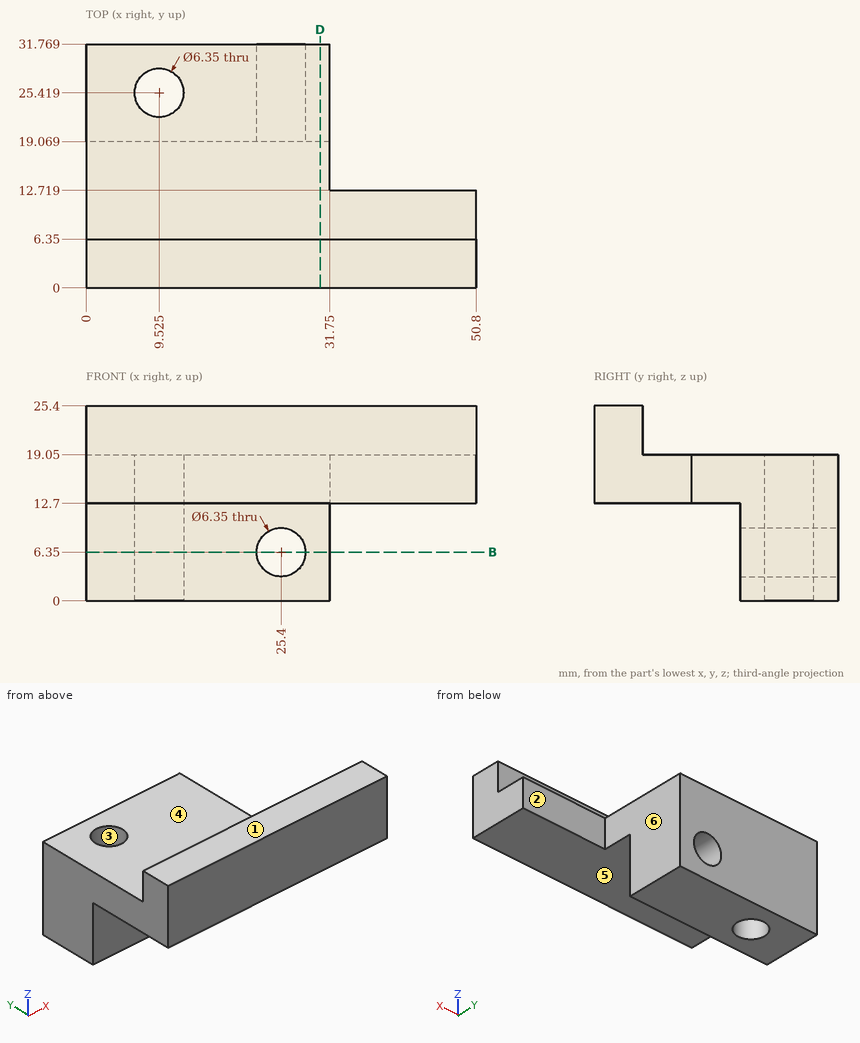
Check sheet for the drawn part. Datum: minimum x, y, z corner. Units: mm. A direction names the side the tool comes from. Give positions to 0.01 mm unless a question says otherwise; leave off trailing zeros. Loops run counter-clockwise (first coordinate to the right, second up) from the corner with the lowest first, then second, coordinate; pieces in that order, holes last. Notation, with made-up numbers: (30, -38) - (58, -38) arc R35 ccw to (58, -6) - close; hole circle Ø4 at (-36.5, 32.25). An arc over 180 degrees is marked (long way). Write each question's results on one line, items separated by ' | '.
1) Depth check by flat-ended pin: P1, Ø3, axis at x = 10.5, y = 25.5, coming from the +Z side; P2, Ø4, axis at x = 13.5, z = 2.5, coming from the -Y side; P3, Ø15.5, axis at x = 19.5, y = 8, coming from the -Z side; P4, Ø7, axis at x = 30, z = 23, coming from the +Y side. Enter the tip coordinate at first touch or a pass-through.
Solution:
P1: through | P2: y = 19.07 | P3: z = 12.7 | P4: y = 6.35
2) Sectioned sample at B-B on z = 6.35. Count the separate pieces of the cut face and the enclosed holes in it, plus the area to 3 significant figures.
Solution:
separate pieces: 2 | enclosed holes: 1 | area: 291 mm2
3) Tool access check on the marked faces 4, 5 and 6. Record the directions out of +Z, -Z, +X, -X, +Y, -Y that give a thin tool (end or side, any length) a straight path to the whole face; none if there is none.
Solution:
face 4: +Z, +X, -X, +Y | face 5: -Z, +X, -X, -Y | face 6: +Z, -Z, +X, +Y
4) Material ranges on L1, parallel to Z at x = 30.5, y = 19; L2, parallel to Y at x = 31, z = 19.5; L3, parallel to X at y = 22, z = 5.75, recorded low to high. Write a range as from..to.
Solution:
L1: 12.7..19.05 | L2: 0..6.35 | L3: 0..22.28, 28.52..31.75
5) Mould release check, pull along Y, two halves, no side actions. Record for the marked faces 1, 2 and 3: pulls with the +Y half, pulls with the -Y half, needs draft (parallel to the pull), parting line crosses it, or undercut.
Solution:
face 1: needs draft | face 2: pulls with the +Y half | face 3: undercut
6) Sectioned sample at D-D on x = 30.5. Record the boundary of the cut face in (y, z).
Solution:
outline: (0, 12.7) - (19.07, 12.7) - (19.07, 0) - (31.77, 0) - (31.77, 19.05) - (6.35, 19.05) - (6.35, 25.4) - (0, 25.4) - close
